from build123d import *

# Parameters (mm, degrees)
SKETCH1_W           = 30
SKETCH1_H           = 50
BOSS_EXTRUDE1_DEPTH = 10
SKETCH2_R           = 5
BOSS_EXTRUDE2_DEPTH = 10
FILLET1_R           = 10
FILLET2_R           = 10
BOSS_EXTRUDE3_DEPTH = 40


with BuildPart() as part:
    # Sketch1 → Boss-Extrude1 (new body)
    with BuildSketch(Plane(origin=(0, 0, 0), x_dir=(1, 0, 0), z_dir=(0, 1, 0))):
        Rectangle(SKETCH1_W, SKETCH1_H)
    extrude(amount=BOSS_EXTRUDE1_DEPTH)

    # Sketch2 → Boss-Extrude2 (add)
    with BuildSketch(Plane(origin=(0, 10, 0), x_dir=(1, 0, 0), z_dir=(0, 1, 0))):
        with Locations(Location((0, -15, 0), (0, 0, 90))):
            Circle(SKETCH2_R)
    extrude(amount=BOSS_EXTRUDE2_DEPTH)

    # Fillet1
    fillet1_edges = [part.edges().sort_by_distance(p)[0] for p in [
        (-15, 5, -25),
        (15, 5, -25),
    ]]
    fillet(fillet1_edges, radius=FILLET1_R)

    # Fillet2
    fillet2_edges = [part.edges().sort_by_distance(p)[0] for p in [
        (15, 5, 25),
        (-15, 5, 25),
    ]]
    fillet(fillet2_edges, radius=FILLET2_R)

    # Sketch3 → Boss-Extrude3 (add)
    with BuildSketch(Plane.XZ):
        with BuildLine():
            Line((10, 15), (10, 5))
            ThreePointArc((10, 5), (8.535533906, 1.464466094), (5, 0))
            Line((5, 0), (-5, 0))
            ThreePointArc((-5, 0), (-8.535533906, 1.464466094), (-10, 5))
            Line((-10, 5), (-10, 15))
            ThreePointArc((-10, 15), (-8.535533906, 18.535533906), (-5, 20))
            Line((-5, 20), (5, 20))
            ThreePointArc((5, 20), (8.535533906, 18.535533906), (10, 15))
        make_face()
    extrude(amount=BOSS_EXTRUDE3_DEPTH)


solid = part.part
Can you work these out from the model? Positions are in its coordinate system, mm. A direction names the side the tool comes from. Give positions to 0.01 mm unless a question says otherwise; leave off trailing zeros. Order: outer loops, then holes, each group sorted by start corner. A loop starts at its lowest first (then second) coordinate and runs counter-clockwise, first axis right, second up. Notation, with made-up numbers: M -34.5,13 L -18.5,13 A14 ccw -18.5,20 Z; hole C 80.25,30 d11. An arc over 180 degrees is marked long. One line per item, written item: value.
Item 1: Please list where these lines run through material, in increasing order: line 1 (Z direction, x = 4, y = -11.5); line 2 (X direction, y = -28.5, z = 5); line 3 (Y direction, x = 5, z = -17).
Verdict:
line 1: 0 to 20
line 2: -10 to 10
line 3: 0 to 10
Item 2: If we section it at D-D on z = -9: Write out the boundary of the cut face in (x, y).
Verdict:
outline: M -15,0 L 15,0 L 15,10 L -15,10 Z
Item 3: If we section it at A-A on x = 0: Write out the boundary of the cut face in (y, z).
Verdict:
outline: M -40,0 L 0,0 L 0,-25 L 10,-25 L 10,10 L 20,10 L 20,20 L 10,20 L 10,25 L 0,25 L 0,20 L -40,20 Z
Item 4: For faces 1 (the face through (9, -20, 2)), 2 (the face through (-8, -20, 1)), 3 (the face through (10, -20, 10)), which set-ups out of +Z, -Z, +X, -X, +Y, -Y let a thin tool reach every point of the face, with its end or its side?
Verdict:
face 1: -Z, +X, -Y
face 2: -Z, -X, -Y
face 3: +Z, -Z, +X, -Y
Item 5: If we section it at C-C on z = 7: Write out the boundary of the cut face in (x, y), and give its area (3 significant figures).
Verdict:
outline: M -15,0 L -10,0 L -10,-40 L 10,-40 L 10,0 L 15,0 L 15,10 L -15,10 Z
area: 1,100 mm2
Item 6: For pin 1 (10 mm diameter, centred on x = 0, z = -6.5, fed in from +Y); pin 2 (5 mm diameter, centred on x = 1, y = -28, fed in from +Z); pin 3 (3 mm diameter, centred on y = -17, z = 7.5, fed in from +X); pin 4 (5 mm diameter, centred on y = -1, z = -8, fed in from -X), each with a flat end and sliding along its axis, tell me the tip position at first contact or that it passes through.
Verdict:
pin 1: y = 10
pin 2: z = 20
pin 3: x = 10
pin 4: x = -15
Item 7: If we section it at B-B on y = -25.5: Write out the boundary of the cut face in (x, z), and give its area (3 significant figures).
Verdict:
outline: M -10,5 A5 ccw -5,0 L 5,0 A5 ccw 10,5 L 10,15 A5 ccw 5,20 L -5,20 A5 ccw -10,15 Z
area: 379 mm2
